Model file for the job. Use its own axes, mm. A direction names the side the tool comes from. Round coordinates to 2 decimals unless told otherwise and drop trailing zeros. Order: outer loops, then holes, each group sorted by start corner. A loop starts at its lowest first (then second) coordinate and runs counter-clockwise, first axis right, second up. Notation, with made-up numbers: (56, 53) -> (79, 53) arc R28 cw to (79, 77) -> close; hole circle Ø5 at (18.5, -6.5). An arc over 180 degrees is marked (long way). Put each result on its own line as item: value. Start each with the question number.
Q1. Cut at D-D, the plane z = 17.5. List the corners of the cut face in (x, y), and give its area (3 significant figures).
Q2. Pull direction Y, two halves, no side cores. Call faces 4 (the face through (-47, 7, 0)), 5 (the face through (-60, 15, 0)), 6 (the face through (-1, 30, 13)): released by +Y, released by -Y, zero draft, split by the parting line, or undercut.
Q3. 3-axis set-ups, long thin cutter, end or side, ignore diameter. For faces 1 (the face through (11.86, 10.14, -22.09)), 2 (the face through (0.49, 13.944, -7.705)), 3 (the face through (0, 20, -22)): which of +Z, -Z, +X, -X, +Y, -Y reach the whole face in a straight line?
Q4. Cut at B-B, the plane y = 13.75. List the corners of the cut face in (x, z), and give its area (3 significant figures).
Q5. Cut at C-C, the plane y = 23. List the corners of the cut face in (x, z), and give its area (3 significant figures).
Q6. Cut at A-A, the plane x = -50. List the corners of the cut face in (y, z).
Q7. Flat gauge pins, fed straight in: P1, Ø6, axis at x = -11, z = -10.5, coming from the +Y side; P2, Ø5, axis at x = 3, z = 4.5, coming from the +Y side. Where does each tip first touch, or does it go through?
Q8. Probe L1, parallel to Y at x = 50, z = 7.5; L2, parallel to Z at x = 0, y = 12.5; L3, parallel to X at y = 13, z = -22. List the from-to ranges inside material, lowest first.
from build123d import *

# Parameters (mm, degrees)
ESQUISSE1_W             = 120
ESQUISSE1_H             = 60
BOSS_EXTRU_1_DEPTH      = 10
BOSS_EXTRU_2_DEPTH      = 20
BOSS_EXTRU_3_DEPTH      = 10
CHANFREIN1_SIZE         = 2
ENL_V_MAT_EXTRU_1_REACH = 62
ESQUISSE4_R             = 3
ENL_V_MAT_EXTRU_2_REACH = 22
ESQUISSE5_R             = 2


with BuildPart() as part:
    # Esquisse1 → Boss.-Extru.1 (new body)
    with BuildSketch(Plane(origin=(0, 0, 0), x_dir=(1, 0, 0), z_dir=(0, 1, 0))):
        Rectangle(ESQUISSE1_W, ESQUISSE1_H)
    extrude(amount=BOSS_EXTRU_1_DEPTH)

    # Esquisse2 → Boss.-Extru.2 (add)
    with BuildSketch(Plane(origin=(0, 10, 0), x_dir=(1, 0, 0), z_dir=(0, 1, 0))):
        with BuildLine():
            Line((-40, 30), (-60, 30))
            Line((-60, 30), (-60, -30))
            Line((-60, -30), (60, -30))
            Line((60, -30), (60, 30))
            Line((60, 30), (40, 30))
            ThreePointArc((40, 30), (0, -10), (-40, 30))
        make_face()
    extrude(amount=BOSS_EXTRU_2_DEPTH)

    # Esquisse3 → Boss.-Extru.3 (add)
    with BuildSketch(Plane(origin=(0, 10, 0), x_dir=(1, 0, 0), z_dir=(0, 1, 0))):
        with BuildLine():
            Line((-22.3, 30), (22.3, 30))
            ThreePointArc((22.3, 30), (0, 7.7), (-22.3, 30))
        make_face()
    extrude(amount=BOSS_EXTRU_3_DEPTH)

    # Chanfrein1
    chanfrein1_edges = [part.edges().sort_by_distance(p)[0] for p in [
        (0, 20, -7.7),
    ]]
    chamfer(chanfrein1_edges, length=CHANFREIN1_SIZE)

    # Esquisse4 → Enlèv. mat.-Extru.1 (cut, up to next)
    with BuildSketch(Plane(origin=(0, 0, -30), x_dir=(-1, 0, 0), z_dir=(0, 0, -1)), mode=Mode.PRIVATE) as enl_v_mat_extru_1_sk1:
        with Locations((-50, 23)):
            Circle(ESQUISSE4_R)
    enl_v_mat_extru_1_tool1 = extrude(enl_v_mat_extru_1_sk1.sketch, amount=-ENL_V_MAT_EXTRU_1_REACH, mode=Mode.PRIVATE) & part.part
    add(enl_v_mat_extru_1_tool1.solids().sort_by_distance((50, 23, -30))[0], mode=Mode.SUBTRACT)
    # Esquisse4 → Enlèv. mat.-Extru.1 (cut, up to next)
    with BuildSketch(Plane(origin=(0, 0, -30), x_dir=(-1, 0, 0), z_dir=(0, 0, -1)), mode=Mode.PRIVATE) as enl_v_mat_extru_1_sk2:
        with Locations((50, 23)):
            Circle(ESQUISSE4_R)
    enl_v_mat_extru_1_tool2 = extrude(enl_v_mat_extru_1_sk2.sketch, amount=-ENL_V_MAT_EXTRU_1_REACH, mode=Mode.PRIVATE) & part.part
    add(enl_v_mat_extru_1_tool2.solids().sort_by_distance((-50, 23, -30))[0], mode=Mode.SUBTRACT)
    # Esquisse4 → Enlèv. mat.-Extru.1 (cut, up to next)
    with BuildSketch(Plane(origin=(0, 0, -30), x_dir=(-1, 0, 0), z_dir=(0, 0, -1)), mode=Mode.PRIVATE) as enl_v_mat_extru_1_sk3:
        with Locations((-50, 7)):
            Circle(ESQUISSE4_R)
    enl_v_mat_extru_1_tool3 = extrude(enl_v_mat_extru_1_sk3.sketch, amount=-ENL_V_MAT_EXTRU_1_REACH, mode=Mode.PRIVATE) & part.part
    add(enl_v_mat_extru_1_tool3.solids().sort_by_distance((50, 7, -30))[0], mode=Mode.SUBTRACT)
    # Esquisse4 → Enlèv. mat.-Extru.1 (cut, up to next)
    with BuildSketch(Plane(origin=(0, 0, -30), x_dir=(-1, 0, 0), z_dir=(0, 0, -1)), mode=Mode.PRIVATE) as enl_v_mat_extru_1_sk4:
        with Locations((50, 7)):
            Circle(ESQUISSE4_R)
    enl_v_mat_extru_1_tool4 = extrude(enl_v_mat_extru_1_sk4.sketch, amount=-ENL_V_MAT_EXTRU_1_REACH, mode=Mode.PRIVATE) & part.part
    add(enl_v_mat_extru_1_tool4.solids().sort_by_distance((-50, 7, -30))[0], mode=Mode.SUBTRACT)

    # Esquisse5 → Enlèv. mat.-Extru.2 (cut, up to next)
    with BuildSketch(Plane(origin=(0, 20, 0), x_dir=(1, 0, 0), z_dir=(0, 1, 0)), mode=Mode.PRIVATE) as enl_v_mat_extru_2_sk1:
        with Locations((0, 14)):
            Circle(ESQUISSE5_R)
    enl_v_mat_extru_2_tool1 = extrude(enl_v_mat_extru_2_sk1.sketch, amount=-ENL_V_MAT_EXTRU_2_REACH, mode=Mode.PRIVATE) & part.part
    add(enl_v_mat_extru_2_tool1.solids().sort_by_distance((0, 20, -14))[0], mode=Mode.SUBTRACT)
    # Esquisse5 → Enlèv. mat.-Extru.2 (cut, up to next)
    with BuildSketch(Plane(origin=(0, 20, 0), x_dir=(1, 0, 0), z_dir=(0, 1, 0)), mode=Mode.PRIVATE) as enl_v_mat_extru_2_sk2:
        with Locations((-13.856406461, 22)):
            Circle(ESQUISSE5_R)
    enl_v_mat_extru_2_tool2 = extrude(enl_v_mat_extru_2_sk2.sketch, amount=-ENL_V_MAT_EXTRU_2_REACH, mode=Mode.PRIVATE) & part.part
    add(enl_v_mat_extru_2_tool2.solids().sort_by_distance((-13.856406, 20, -22))[0], mode=Mode.SUBTRACT)
    # Esquisse5 → Enlèv. mat.-Extru.2 (cut, up to next)
    with BuildSketch(Plane(origin=(0, 20, 0), x_dir=(1, 0, 0), z_dir=(0, 1, 0)), mode=Mode.PRIVATE) as enl_v_mat_extru_2_sk3:
        with Locations((13.856406461, 22)):
            Circle(ESQUISSE5_R)
    enl_v_mat_extru_2_tool3 = extrude(enl_v_mat_extru_2_sk3.sketch, amount=-ENL_V_MAT_EXTRU_2_REACH, mode=Mode.PRIVATE) & part.part
    add(enl_v_mat_extru_2_tool3.solids().sort_by_distance((13.856406, 20, -22))[0], mode=Mode.SUBTRACT)


solid = part.part
Ans:
1. outline: (-60, 0) -> (60, 0) -> (60, 30) -> (-60, 30) -> close; hole circle Ø6 at (-50, 7); hole circle Ø6 at (-50, 23); hole circle Ø6 at (50, 7); hole circle Ø6 at (50, 23)
1. area: 3,490 mm^2
2. face 4: undercut
2. face 5: zero draft
2. face 6: released by +Y
3. face 1: +Y, -Y
3. face 2: +Y
3. face 3: -Z, +Y
4. outline: (-60, -30) -> (-40, -30) arc R40 cw to (40, -30) -> (60, -30) -> (60, 30) -> (-60, 30) -> close; (-22.3, -30) -> (22.3, -30) arc R22.3 ccw to start; hole circle Ø4 at (-13.86, -22); hole circle Ø4 at (0, -14); hole circle Ø4 at (13.86, -22)
4. area: 5,430 mm^2
5. outline: (-60, -30) -> (-53, -30) -> (-53, 30) -> (-60, 30) -> close; (-47, -30) -> (-40, -30) arc R40 cw to (40, -30) -> (47, -30) -> (47, 30) -> (-47, 30) -> close; (53, -30) -> (60, -30) -> (60, 30) -> (53, 30) -> close
5. area: 3,970 mm^2
6. outline: (0, -30) -> (4, -30) -> (4, 30) -> (0, 30) -> close; (10, -30) -> (20, -30) -> (20, 30) -> (10, 30) -> close; (26, -30) -> (30, -30) -> (30, 30) -> (26, 30) -> close
7. P1: stops at y = 20
7. P2: stops at y = 10
8. L1: y = 0 to 4, 10 to 20, 26 to 30
8. L2: z = -30 to -16, -12 to -7.7, 10 to 30
8. L3: x = -60 to -39.19, -20.82 to -15.86, -11.86 to 11.86, 15.86 to 20.82, 39.19 to 60
